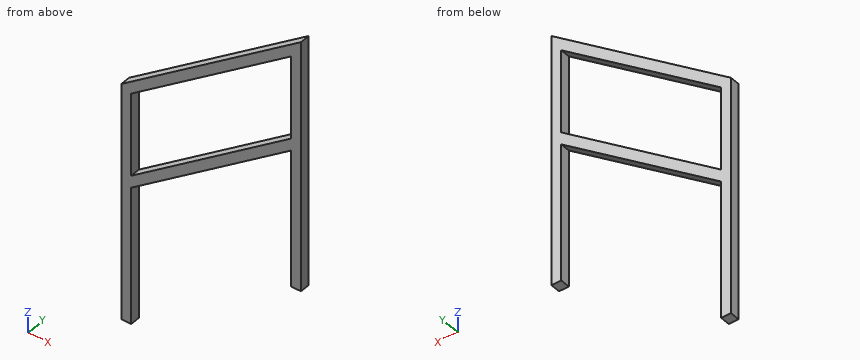
```python
from build123d import *

# Parameters (mm, degrees)
F1_DEPTH = 44.45


with BuildPart() as f1:
    # F0 (on Front) → F1 (new body)
    with BuildSketch(Plane.XZ):
        Polygon((44.45, -399.401926), (44.45, -454.345147), (768.35, 71.598989), (768.35, 126.54221), align=None)
        Polygon((812.8, 590.533767), (0, 0), (0, -1079.5), (44.45, -1079.5), (44.45, -454.345147), (44.45, -399.401926), (44.45, -22.648406), (768.35, 503.29573), (768.35, 126.54221), (768.35, 71.598989), (768.35, -552.466233), (812.8, -552.466233), align=None)
    extrude(amount=F1_DEPTH)


solid = f1.part
```
Geometry: final body of the model. Coordinates: model frame, mm. Coordinates: 2 decimals unless noted, no trailing zeros. Order: outer loops, then holes, each group sorted by start corner. A loop starts at its lowest first (then second) coordinate and runs counter-clockwise, first axis right, second up. Notation, with made-up numbers: M -33,69 L 26,69 A12 ccw 26,90 Z; hole C 33.25,69 d1. An arc over 180 degrees is marked long. Answer in a Markdown table with one row per item. Add a question column.
Q1. Contact query for flat-ended pins moving along their axis: P1, Ø4, axis at y = -39, z = 336, coming from the -X side; P2, Ø1.5, axis at y = -20, z = -687, coming from the +X side; P3, Ø4, axis at x = 639.5, y = -28.5, coming from the -Z side. Output: stop coordinate, or through.
Q2. Section query A-A on y = -24. Return the cut outline in (x, z).
Q3. Section query B-B on x = 656. Return the cut outline in (y, z), and give its area (3 significant figures).
Q4. Section query D-D on z = 255. Return the cut outline in (x, y), and give its area (3 significant figures).
Q5. Section query C-C on z = -87. Return the cut outline in (x, y), and give its area (3 significant figures).
Q6. Line query: L1, parallel to X at y = -16.5, z = -524.5; L2, parallel to X at y = -5, z = -262; L3, parallel to X at y = -10, z = -27. Output: solid intervals per line, ascending.
Completed:
| question | item | result |
|---|---|---|
| 1 | P1 | stops at x = 459.71 |
| 1 | P2 | stops at x = 44.45 |
| 1 | P3 | stops at z = -23.47 |
| 2 | outline | M 0,-1079.5 L 44.45,-1079.5 L 44.45,-454.35 L 768.35,71.6 L 768.35,-552.47 L 812.8,-552.47 L 812.8,590.53 L 0,0 Z; hole M 44.45,-399.4 L 768.35,126.54 L 768.35,503.3 L 44.45,-22.65 Z |
| 3 | outline | M -44.45,-10.03 L 0,-10.03 L 0,44.92 L -44.45,44.92 Z; M -44.45,421.67 L 0,421.67 L 0,476.61 L -44.45,476.61 Z |
| 3 | area | 4,880 mm2 |
| 4 | outline | M 350.98,-44.45 L 426.6,-44.45 L 426.6,0 L 350.98,0 Z; M 768.35,-44.45 L 812.8,-44.45 L 812.8,0 L 768.35,0 Z |
| 4 | area | 5,340 mm2 |
| 5 | outline | M 0,-44.45 L 44.45,-44.45 L 44.45,0 L 0,0 Z; M 474.43,-44.45 L 550.06,-44.45 L 550.06,0 L 474.43,0 Z; M 768.35,-44.45 L 812.8,-44.45 L 812.8,0 L 768.35,0 Z |
| 5 | area | 7,310 mm2 |
| 6 | L1 | x = 0 to 44.45, 768.35 to 812.8 |
| 6 | L2 | x = 0 to 44.45, 233.57 to 309.19, 768.35 to 812.8 |
| 6 | L3 | x = 0 to 44.45, 557.02 to 632.64, 768.35 to 812.8 |
